Part print with two shaded views. Sizes in mm from the minimum x, y, z corner. A direction names the side the tool comes from. Give positions to 0.01 mm unless a question says otherwise; leave off trailing zeros. Write each loop counter-clockwise with the first axis right and the second up, starting at its lowest first coordinate (ties: lowest second). Pieces come first, ordered by that corner, then holes. Notation, with made-up numbers: (13, 12) -> (64, 12) arc R24 cw to (64, 39) -> close; hole circle Ø9 at (35, -34.75). An arc over 180 degrees is marked (long way). Write item = value, one per line. Start each with the question number.
Q1. Drop flat-ended pins along their axis: P1, Ø8, axis at x = 35, z = 10, coming from the -Y side; P2, Ø10, axis at x = 26, z = 34, coming from the +Y side; P3, Ø8.5, axis at x = 27.5, y = 30.5, coming from the +Z side; P4, Ø1, axis at y = 12, z = 15.5, coming from the -X side. Give the stop position or say it passes through.
Q2. Mould opens along Z. For the marked faces 4, 5 and 6 say: pulls with the +Z half, pulls with the -Z half, needs draft (parallel to the pull), parting line crosses it, or undercut.
Q3. Saw through at B-B, the plane x = 28. List the corners of the cut face in (y, z), then the cut area to 3 significant figures.
Q4. Wall check: line 1 (Z direction, x = 35, y = 32.5); line 2 (X direction, y = 3, z = 10); line 3 (Y direction, x = 27.5, z = 5). Give the ranges that are in metal, low to high.
Q5. Saw through at A-A, the plane y = 22. List the corners of the cut face in (x, z), then the cut area to 3 significant figures.
Q6. Saw through at C-C, the plane z = 16.5. List the corners of the cut face in (x, y).
Q7. Saw through at D-D, the plane x = 35. List the corners of the cut face in (y, z).
Q8. Tool access for the marked faces 1, 2 and 3: list every direction of +Z, -Z, +X, -X, +Y, -Y with a clear straight run to the whole face (end or side of a thin tool).
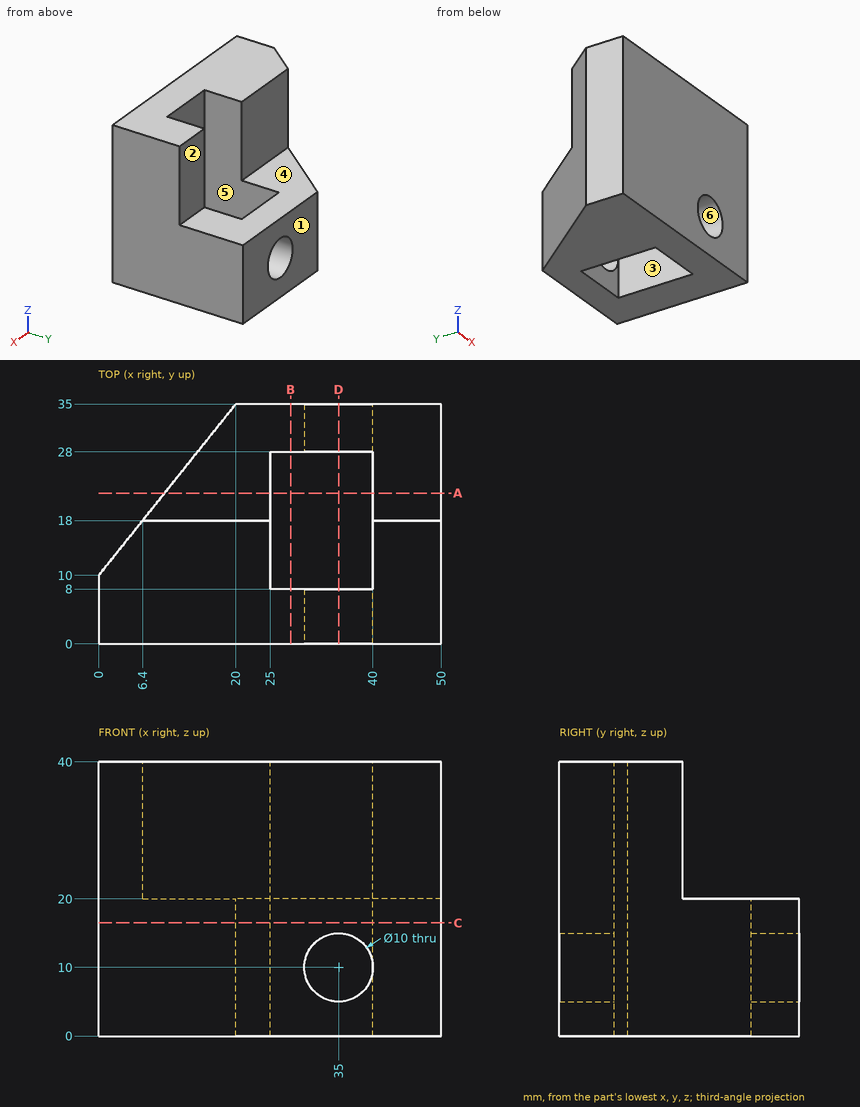
Report:
q1.P1 = through
q1.P2 = 18
q1.P3 = 20
q1.P4 = 1.2
q2.face_4 = pulls with the +Z half
q2.face_5 = needs draft
q2.face_6 = undercut
q3.outline = (0, 0) -> (8, 0) -> (8, 40) -> (0, 40) -> close; (28, 0) -> (35, 0) -> (35, 20) -> (28, 20) -> close
q3.area = 460 mm2
q4.line_1 = 0 to 5, 15 to 20
q4.line_2 = 0 to 30, 40 to 50
q4.line_3 = 0 to 8, 28 to 35
q5.outline = (9.6, 0) -> (25, 0) -> (25, 20) -> (9.6, 20) -> close; (40, 0) -> (50, 0) -> (50, 20) -> (40, 20) -> close
q5.area = 508 mm2
q6.outline = (0, 0) -> (50, 0) -> (50, 35) -> (20, 35) -> (0, 10) -> close; hole (25, 8) -> (40, 8) -> (40, 28) -> (25, 28) -> close
q7.outline = (0, 0) -> (8, 0) -> (8, 5) -> (0, 5) -> close; (0, 15) -> (8, 15) -> (8, 40) -> (0, 40) -> close; (28, 0) -> (35, 0) -> (35, 5) -> (28, 5) -> close; (28, 15) -> (35, 15) -> (35, 20) -> (28, 20) -> close
q8.face_1 = +Z, -Z, +X, -X, +Y
q8.face_2 = +Z, +X, -X, +Y
q8.face_3 = +Z, -Z
